Autodesk Inventor part; units mm, degrees
ref_plane "YZ Plane" through (0, 0, 0) normal (1, 0, 0) x (0, 1, 0)
ref_plane "XZ Plane" through (0, 0, 0) normal (0, 1, 0) x (-1, 0, 0)
ref_plane "XY Plane" through (0, 0, 0) normal (0, 0, 1) x (1, 0, 0)
sketch "スケッチ1" plane through (0, 0, 0) normal (0, 0, 1) x (1, 0, 0)
  line L0 (5, -5) -> (-5, -5)
  line L1 (-5, -5) -> (-5, 5)
  line L2 (-5, 5) -> (5, 5)
  line L3 (5, 5) -> (5, -5)
  line L4 (5, -5) -> (-5, 5) construction
  line L5 (-5, -5) -> (5, 5) construction
  line L6 (4, 4) -> (-4, 4)
  line L7 (-4, 4) -> (-4, -4)
  line L8 (-4, -4) -> (4, -4)
  line L9 (4, -4) -> (4, 4)
  point P0 (0, 0)
  dimension "d0" = 10
  dimension "d1" = 10
  dimension "d2" = 1
extrude "押し出し1" add sketch "スケッチ1" along normal blind 30
sketch "スケッチ2" plane through (5, -5, 0) normal (1, 0, 0) x (0, 0, -1)
  line L0 (-30, 10) -> (-30, 0)
  line L1 (-30, 5) -> (0, 5)
  line L2 (0, 0) -> (0, 10)
  point P0 (-10, 5)
  dimension "d5" = 10
hole "穴1" at (5, 0, 10) direction (-1, 0, 0) diameter 3.3 end through all
sketch "スケッチ3" plane through (-5, 5, 0) normal (0, 1, 0) x (1, 0, 0)
  line L0 (5, 0) -> (5, -30)
  line L1 (1, -30) -> (9, -30)
  line L2 (10, 0) -> (0, 0)
  point P0 (5, -20)
  dimension "d13" = 20
hole "穴2" at (0, 5, 20) direction (0, -1, 0) diameter 3.3 end through all
properties part number "small_kaku_1010_santen"
Geometry check sheet. Reference: the model listing, model coordinates, mm. A direction names the side the tool comes from. Give positions to 0.01 mm unless a question says otherwise; leave off trailing zeros. Write each loop counter-clockwise with the first axis right and the second up, starting at its lowest first coordinate (ties: lowest second). Pieces come first, ordered by that corner, then holes.
1) Section check C-C, the plane z = 10. Record the boundary of the cut face in (x, y).
2) Material ranges on L1, parallel to Y at x = -3.25, z = 20; L2, parallel to Z at x = 4.25, y = 0, recorded low to high.
3) Release check for a two-part mould opening along Y. For faces 3 (the flat face through (-4, 0, 15)), 4 (the flat face through (5, 0, 15)), 5 (the flat face through (4, 0, 15)), 6 (the flat face through (0, 5, 15)) record: pulls with the +Y half, pulls with the -Y half, needs draft (parallel to the pull), parting line crosses it, or undercut.
4) Section check B-B, the plane y = 0. Record the boundary of the cut face in (x, z), and give its area (3 significant figures).
5) Section check D-D, the plane y = 2. Record the boundary of the cut face in (x, z), and give its area (3 significant figures).
6) Section check A-A, the plane x = 0. Record the boundary of the cut face in (y, z), and give its area (3 significant figures).
7) Access from +Z, -Z, +X, -X, +Y, -Y to the whole of each face (thin tool, end or side, straight path). Record for faces 1 (the flat face through (0, -4, 15)), 2 (the cylindrical face through (4.493, 0.632, 8.476)).
Computed:
1. outline: (-5, -5) - (5, -5) - (5, -1.65) - (4, -1.65) - (4, -4) - (-4, -4) - (-4, -1.65) - (-5, -1.65) - close; (-5, 1.65) - (-4, 1.65) - (-4, 4) - (4, 4) - (4, 1.65) - (5, 1.65) - (5, 5) - (-5, 5) - close
2. L1: y = -5 to -4, 4 to 5
2. L2: z = 0 to 8.35, 11.65 to 30
3. face 3: undercut
3. face 4: needs draft
3. face 5: undercut
3. face 6: pulls with the +Y half
4. outline: (-5, 0) - (-4, 0) - (-4, 8.35) - (-5, 8.35) - close; (-5, 11.65) - (-4, 11.65) - (-4, 30) - (-5, 30) - close; (4, 0) - (5, 0) - (5, 8.35) - (4, 8.35) - close; (4, 11.65) - (5, 11.65) - (5, 30) - (4, 30) - close
4. area: 53.4 mm2
5. outline: (-5, 0) - (-4, 0) - (-4, 30) - (-5, 30) - close; (4, 0) - (5, 0) - (5, 30) - (4, 30) - close
5. area: 60.0 mm2
6. outline: (-5, 0) - (-4, 0) - (-4, 18.35) - (-5, 18.35) - close; (-5, 21.65) - (-4, 21.65) - (-4, 30) - (-5, 30) - close; (4, 0) - (5, 0) - (5, 18.35) - (4, 18.35) - close; (4, 21.65) - (5, 21.65) - (5, 30) - (4, 30) - close
6. area: 53.4 mm2
7. face 1: +Z, -Z
7. face 2: +X, -X
